Geometry check sheet. Reference: the model listing, model coordinates, mm. Coordinates: 2 decimals unless noted, no trailing zeros. Loops run counter-clockwise (first coordinate to the right, second up) from the corner with the lowest first, then second, coordinate; pieces in that order, holes last.
from build123d import *

# Parameters (mm, degrees)
F1_DEPTH = 12
F2_SIZE  = 0.5


with BuildPart() as f1:
    # F0 (on Top) → F1 (new body)
    with BuildSketch(Plane.XY):
        with BuildLine():
            Line((-11.60309311, 3.5892210044), (-11.60309311, 5.5892210044))
            ThreePointArc((-11.60309311, 5.5892210044), (-18.10309311, -0.9107789956), (-11.60309311, -7.4107789956))
            Line((-11.60309311, -7.4107789956), (-11.60309311, -5.4107789956))
            ThreePointArc((-11.60309311, -5.4107789956), (-16.10309311, -0.9107789956), (-11.60309311, 3.5892210044))
        make_face()
        with BuildLine():
            ThreePointArc((-5.10309311, -0.9107789956), (-7.0068990323, 3.6854150821), (-11.60309311, 5.5892210044))
            Line((-11.60309311, 5.5892210044), (-11.60309311, 3.5892210044))
            ThreePointArc((-11.60309311, 3.5892210044), (-8.4211125947, 2.2712015197), (-7.10309311, -0.9107789956))
            ThreePointArc((-7.10309311, -0.9107789956), (-8.4211125947, -4.0927595109), (-11.60309311, -5.4107789956))
            Line((-11.60309311, -5.4107789956), (-6.9126773502, -5.4107789956))
            ThreePointArc((-6.9126773502, -5.4107789956), (-5.572433841, -3.3358869892), (-5.10309311, -0.9107789956))
        make_face()
        with BuildLine():
            Line((18.39690689, 5.5892210044), (-11.60309311, 5.5892210044))
            ThreePointArc((-11.60309311, 5.5892210044), (-7.0068990323, 3.6854150821), (-5.10309311, -0.9107789956))
            ThreePointArc((-5.10309311, -0.9107789956), (-5.572433841, -3.3358869892), (-6.9126773502, -5.4107789956))
            Line((-6.9126773502, -5.4107789956), (13.7064911302, -5.4107789956))
            ThreePointArc((13.7064911302, -5.4107789956), (12.4177765184, 1.6387307612), (18.39690689, 5.5892210044))
        make_face()
        with BuildLine():
            Line((18.39690689, 3.5892210044), (18.39690689, 5.5892210044))
            ThreePointArc((18.39690689, 5.5892210044), (12.4177765184, 1.6387307612), (13.7064911302, -5.4107789956))
            Line((13.7064911302, -5.4107789956), (18.39690689, -5.4107789956))
            ThreePointArc((18.39690689, -5.4107789956), (13.89690689, -0.9107789956), (18.39690689, 3.5892210044))
        make_face()
        with BuildLine():
            ThreePointArc((24.89690689, -0.9107789956), (22.9931009677, 3.6854150821), (18.39690689, 5.5892210044))
            Line((18.39690689, 5.5892210044), (18.39690689, 3.5892210044))
            ThreePointArc((18.39690689, 3.5892210044), (21.5788874053, 2.2712015197), (22.89690689, -0.9107789956))
            ThreePointArc((22.89690689, -0.9107789956), (21.5788874053, -4.0927595109), (18.39690689, -5.4107789956))
            Line((18.39690689, -5.4107789956), (18.39690689, -7.4107789956))
            ThreePointArc((18.39690689, -7.4107789956), (22.9931009677, -5.5069730733), (24.89690689, -0.9107789956))
        make_face()
        with BuildLine():
            Line((18.39690689, -5.4107789956), (13.7064911302, -5.4107789956))
            ThreePointArc((13.7064911302, -5.4107789956), (15.8473971332, -6.8899093672), (18.39690689, -7.4107789956))
            Line((18.39690689, -7.4107789956), (18.39690689, -5.4107789956))
        make_face()
        with BuildLine():
            ThreePointArc((-6.9126773502, -5.4107789956), (-9.0535833532, -6.8899093672), (-11.60309311, -7.4107789956))
            Line((-11.60309311, -7.4107789956), (18.39690689, -7.4107789956))
            ThreePointArc((18.39690689, -7.4107789956), (15.8473971332, -6.8899093672), (13.7064911302, -5.4107789956))
            Line((13.7064911302, -5.4107789956), (-6.9126773502, -5.4107789956))
        make_face()
        with BuildLine():
            Line((-11.60309311, -5.4107789956), (-11.60309311, -7.4107789956))
            ThreePointArc((-11.60309311, -7.4107789956), (-9.0535833532, -6.8899093672), (-6.9126773502, -5.4107789956))
            Line((-6.9126773502, -5.4107789956), (-11.60309311, -5.4107789956))
        make_face()
    extrude(amount=F1_DEPTH)

    # F2
    f2_edges = [f1.edges().sort_by_distance(p)[0] for p in [
        (-18.103093, -0.910779, 12),
        (3.396907, -7.410779, 12),
        (24.896907, -0.910779, 12),
        (3.396907, 5.589221, 12),
        (-11.603093, 3.589221, 12),
        (18.396907, 3.589221, 12),
        (-18.103093, -0.910779, 0),
        (3.396907, -7.410779, 0),
        (24.896907, -0.910779, 0),
        (3.396907, 5.589221, 0),
        (-11.603093, 3.589221, 0),
        (18.396907, 3.589221, 0),
    ]]
    chamfer(f2_edges, length=F2_SIZE)


with BuildPart() as f3_1:
    # F3: copy of F1
    add(f1.part.moved(Location((0, -24.4623, 0))))


solid = f1.part
1) Section check B-B on y = -0.25. Count the separate pieces of the cut face and the enclosed holes in it, and give its area (3 significant figures).
Data:
separate pieces: 3
enclosed holes: 0
area: 300 mm2
2) Material ranges on probe 1 along X at (y, z) = (2.25, 11); probe 2 along X at (y, z) = (1.75, 5.25); probe 3 along Y at (x, z) = (-9.5, 8.5), recorded low to high.
Data:
probe 1: x = -17.28 to -14.81, -8.4 to 15.19, 21.6 to 24.08
probe 2: x = -17.53 to -15.23, -7.97 to 14.77, 22.03 to 24.33
probe 3: y = -7.41 to -4.89, 3.07 to 5.59
3) Depth check by flat-ended pin: pin 1 (6 mm diameter, centred on y = -5.5, z = 3, fed in from +X); pin 2 (2 mm diameter, centred on x = 6.5, y = 1, fed in from -Z). Enter the tip coordinate at first touch or a pass-through.
Data:
pin 1: stops at x = 24.7
pin 2: stops at z = 0
4) Section check A-A on z = 8. Record the cut outline in (x, y).
Data:
outline: (-11.6, -7.41) - (18.4, -7.41) arc R6.5 ccw to (18.4, 5.59) - (-11.6, 5.59) arc R6.5 ccw to start; hole circle Ø9 at (-11.6, -0.91); hole circle Ø9 at (18.4, -0.91)
